Check sheet for the modelled part. Datum: model origin and axes. Units: mm. A direction names the side the tool comes from. Coordinates: 2 decimals unless noted, no trailing zeros. Loops run counter-clockwise (first coordinate to the right, second up) from the corner with the lowest first, then second, coordinate; pieces in that order, holes last.
```python
from build123d import *
from OCP.BRepFilletAPI import BRepFilletAPI_MakeChamfer

# Parameters (mm, degrees)
SKETCH1_W           = 215
SKETCH1_H           = 76.1
SKETCH1_R           = 2.65
BOSS_EXTRUDE1_DEPTH = 10
SKETCH2_W           = 19.75
SKETCH2_H           = 9.75
CUT_EXTRUDE1_DEPTH  = 115.472933482
CHAMFER1_SIZE       = 10
CHAMFER1_SIZE2      = 17.320508076
SKETCH3_R           = 2
CUT_EXTRUDE2_DEPTH  = 115.472933482


with BuildPart() as part:
    # Sketch1 → Boss-Extrude1 (new body)
    with BuildSketch(Plane(origin=(0, 0, 0), x_dir=(1, 0, 0), z_dir=(0, 1, 0))):
        Rectangle(SKETCH1_W, SKETCH1_H)
        with Locations(Location((-40.15, 26.05, 0), (0, 0, 270))):
            Circle(SKETCH1_R, mode=Mode.SUBTRACT)
        with Locations(Location((40.15, 26.05, 0), (0, 0, 90))):
            Circle(SKETCH1_R, mode=Mode.SUBTRACT)
        with Locations(Location((0, 26.05, 0), (0, 0, 270))):
            Circle(SKETCH1_R, mode=Mode.SUBTRACT)
        with Locations(Location((-28.15, -26.05, 0), (0, 0, 270))):
            Circle(SKETCH1_R, mode=Mode.SUBTRACT)
        with Locations(Location((28.15, -26.05, 0), (0, 0, 90))):
            Circle(SKETCH1_R, mode=Mode.SUBTRACT)
    extrude(amount=BOSS_EXTRUDE1_DEPTH)

    # Sketch2 → Cut-Extrude1 (cut, through all)
    with BuildSketch(Plane(origin=(0, 10, 0), x_dir=(1, 0, 0), z_dir=(0, 1, 0))):
        with Locations((-77.35, -15)):
            Rectangle(SKETCH2_W, SKETCH2_H)
        with Locations((-77.35, 15)):
            Rectangle(SKETCH2_W, SKETCH2_H)
        with Locations((77.35, 15)):
            Rectangle(SKETCH2_W, SKETCH2_H)
        with Locations((77.35, -15)):
            Rectangle(SKETCH2_W, SKETCH2_H)
    extrude(amount=-CUT_EXTRUDE1_DEPTH, mode=Mode.SUBTRACT)

    # Chamfer1: one chamfer whose edges measure the first distance from different faces: ONE call of the kernel's chamfer builder (chamfer() names one face for all edges)
    chamfer1_edges_1 = [part.edges().sort_by_distance(p)[0] for p in [
        (-107.5, 5, -38.05),
        (-107.5, 5, 38.05),
    ]]
    chamfer1_side_1 = [part.faces().sort_by_distance(p)[0] for p in [
        (-107.5, 5, 0),
    ]]
    chamfer1_edges_2 = [part.edges().sort_by_distance(p)[0] for p in [
        (107.5, 5, -38.05),
        (107.5, 5, 38.05),
    ]]
    chamfer1_side_2 = [part.faces().sort_by_distance(p)[0] for p in [
        (107.5, 5, 0),
    ]]
    chamfer1 = BRepFilletAPI_MakeChamfer(part.part.solid().wrapped)
    for e in chamfer1_edges_1:
        chamfer1.Add(CHAMFER1_SIZE, CHAMFER1_SIZE2, e.wrapped, chamfer1_side_1[0].wrapped)  # the first distance lies on this face
    for e in chamfer1_edges_2:
        chamfer1.Add(CHAMFER1_SIZE, CHAMFER1_SIZE2, e.wrapped, chamfer1_side_2[0].wrapped)  # the first distance lies on this face
    add(Compound.cast(chamfer1.Shape()), mode=Mode.REPLACE)

    # Sketch3 → Cut-Extrude2 (cut, through all)
    with BuildSketch(Plane(origin=(0, 10, 0), x_dir=(1, 0, 0), z_dir=(0, 1, 0))):
        with Locations(Location((-55, -30, 0), (0, 0, 270))):
            Circle(SKETCH3_R)
        with Locations(Location((-55, 30, 0), (0, 0, 90))):
            Circle(SKETCH3_R)
        with Locations(Location((55, -30, 0), (0, 0, 90))):
            Circle(SKETCH3_R)
        with Locations(Location((55, 30, 0), (0, 0, 270))):
            Circle(SKETCH3_R)
    extrude(amount=-CUT_EXTRUDE2_DEPTH, mode=Mode.SUBTRACT)


solid = part.part
```
1) Section check B-B on x = 40.15. Enter the section's corners in (y, z).
Answer sheet:
outline: (0, -38.05) - (10, -38.05) - (10, -28.7) - (0, -28.7) - close; (0, -23.4) - (10, -23.4) - (10, 38.05) - (0, 38.05) - close
2) Section check D-D on z = 26.05. Enter the section's corners in (x, y), plus the area to 3 significant figures.
Answer sheet:
outline: (-107.5, 0) - (-30.8, 0) - (-30.8, 10) - (-107.5, 10) - close; (-25.5, 0) - (25.5, 0) - (25.5, 10) - (-25.5, 10) - close; (30.8, 0) - (107.5, 0) - (107.5, 10) - (30.8, 10) - close
area: 2,040 mm2
3) Set-up check for faces 1 (the flat face through (-1, 5, 38.05)), 2 (the flat face through (-87.225, 5, 15)): record each of +Z, -Z, +X, -X, +Y, -Y from which the full face is reachable in a straight line by a thin tool's end or side.
Answer sheet:
face 1: +Z, +X, -X, +Y, -Y
face 2: +Y, -Y
4) Section check C-C on y = 2.5. Give the number of separate pieces and of enclosed holes in the cut face, plus the area to 3 significant figures.
Answer sheet:
separate pieces: 1
enclosed holes: 13
area: 15,100 mm2
5) Depth check by flat-ended pin: pin 1 (2.5 mm diameter, centred on x = -55, z = -30, fed in from -Y). Enter the tip coordinate at first touch or a pass-through.
Answer sheet:
pin 1: passes through
6) Scan lines: line 1 (X direction, y = 1.25, z = 17) (3 decimals); line 2 (X direction, y = 4.25, z = 26.05); line 3 (X direction, y = 5.5, z = -26.05). Record each from-to range of solid material in increasing order.
Answer sheet:
line 1: x = -107.5 to -87.225, -67.475 to 67.475, 87.225 to 107.5
line 2: x = -107.5 to -30.8, -25.5 to 25.5, 30.8 to 107.5
line 3: x = -107.5 to -42.8, -37.5 to -2.65, 2.65 to 37.5, 42.8 to 107.5
7) Section check A-A on z = -26.05. Enter the section's corners in (x, y).
Answer sheet:
outline: (-107.5, 0) - (-42.8, 0) - (-42.8, 10) - (-107.5, 10) - close; (-37.5, 0) - (-2.65, 0) - (-2.65, 10) - (-37.5, 10) - close; (2.65, 0) - (37.5, 0) - (37.5, 10) - (2.65, 10) - close; (42.8, 0) - (107.5, 0) - (107.5, 10) - (42.8, 10) - close
8) Mould release check, pull along X, two halves, no side actions. Record for faces 3 (the flat face through (-1, 5, -38.05)), 4 (the flat face through (-107.5, 5, 0)), 5 (the cylindrical face through (25.52, 4.93, 26.39)): +X half, -X half, draft (parallel to the pull), parting line (faces both ways), or undercut.
Answer sheet:
face 3: draft
face 4: -X half
face 5: undercut
